Geometry check sheet. Reference: the model listing, model coordinates, mm. A direction names the side the tool comes from. Give positions to 0.01 mm unless a question says otherwise; leave off trailing zeros. Write each loop counter-clockwise with the first axis right and the second up, starting at its lowest first coordinate (ties: lowest second). Pieces come first, ordered by that corner, then holes. Notation, with made-up numbers: (-7, 62) -> (52, 62) arc R24 cw to (52, 80) -> close; hole circle Ø9 at (-7.75, 58). An arc over 180 degrees is marked (long way). One line per item, written item: value.
Autodesk Inventor part; units mm, degrees
ref_plane "YZ Plane" through (0, 0, 0) normal (1, 0, 0) x (0, 1, 0)
ref_plane "XZ Plane" through (0, 0, 0) normal (0, 1, 0) x (-1, 0, 0)
ref_plane "XY Plane" through (0, 0, 0) normal (0, 0, 1) x (1, 0, 0)
sketch "Sketch1" plane through (0, 0, 0) normal (0, 1, 0) x (-1, 0, 0)
  circle A0 centre (0, 0) radius 5
  dimension "d0" = 10
extrude "Extrusion1" add sketch "Sketch1" along normal blind 23
sketch "Sketch2" plane through (0, 23, 0) normal (0, 1, 0) x (1, 0, 0)
  line L0 (0, -4.5) -> (0, 4.5) construction
  circle A0 centre (0, 0) radius 5
  line L1 (-2.1794, -4.5) -> (2.1794, -4.5)
  line L2 (-2.1794, 4.5) -> (2.1794, 4.5)
extrude "Extrusion2" cut sketch "Sketch2" against normal blind 10 contours L2 A0 | A0 L1
sketch "Sketch3" plane through (0, 23, 0) normal (0, 1, 0) x (1, 0, 0)
  circle A0 centre (0, 0) radius 2.5
  dimension "d7" = 5
extrude "Extrusion3" add sketch "Sketch3" along normal blind 22
sketch "Sketch4" plane through (0, 0, 0) normal (0, -1, 0) x (1, 0, 0)
  circle A0 centre (0, 0) radius 2.5
  circle A1 centre (0, 0) radius 3
  dimension "d10" = 6
extrude "Extrusion4" add sketch "Sketch4" along normal blind 20 contours A0
thread "Thread1"
fillet "Fillet1" radius 0.5 1 edges at (-2.5, 45, 0)
thread "Thread2"
fillet "Fillet2" radius 0.5 1 edges at (-2.5, -20, 0)
properties part number "Semi alberto M"
1) Sectioned sample at B-B on z = 0. Record the cut outline in (x, y).
Verdict:
outline: (-5, 0) -> (-2.5, 0) -> (-2.5, -19.5) arc R0.5 ccw to (-2, -20) -> (2, -20) arc R0.5 ccw to (2.5, -19.5) -> (2.5, 0) -> (5, 0) -> (5, 23) -> (2.5, 23) -> (2.5, 44.5) arc R0.5 ccw to (2, 45) -> (-2, 45) arc R0.5 ccw to (-2.5, 44.5) -> (-2.5, 23) -> (-5, 23) -> close
2) Sectioned sample at C-C on y = 27. Record the cut outline in (x, z), plus the area to 3 significant figures.
Verdict:
outline: circle Ø5 at (0, 0)
area: 19.6 mm^2
3) Depth check by flat-ended pin: pin 1 Ø4 at (y, z) = (5, 3) entering from +X; pin 2 Ø1.3 at (x, y) = (0, 18) entering from -Z; pin 3 Ø2 at (y, z) = (10.5, 3.5) entering from -X. Enter the tip coordinate at first touch or a pass-through.
Verdict:
pin 1: x = 4.9
pin 2: z = -4.5
pin 3: x = -4.33
4) Tool access check on faces 1 (the flat face through (0, 18, 4.5)), 2 (the cylindrical face through (-4.619, 11.339, 1.915)), 3 (the flat face through (0, 18, -4.5)), 4 (the flat face through (2, 23, 2)), 5 (the cylindrical face through (-0.54, -9.61, 2.44)). Record the directions out of +Z, -Z, +X, -X, +Y, -Y that give a thin tool (end or side, any length) a straight path to the whole face; none if there is none.
Verdict:
face 1: +Z, +X, -X, +Y
face 2: +Y, -Y
face 3: -Z, +X, -X, +Y
face 4: +Y
face 5: -Y
5) Sectioned sample at A-A on x = 0. Record the cut outline in (y, z).
Verdict:
outline: (-20, -2) arc R0.5 ccw to (-19.5, -2.5) -> (0, -2.5) -> (0, -5) -> (13, -5) -> (13, -4.5) -> (23, -4.5) -> (23, -2.5) -> (44.5, -2.5) arc R0.5 ccw to (45, -2) -> (45, 2) arc R0.5 ccw to (44.5, 2.5) -> (23, 2.5) -> (23, 4.5) -> (13, 4.5) -> (13, 5) -> (0, 5) -> (0, 2.5) -> (-19.5, 2.5) arc R0.5 ccw to (-20, 2) -> close
6) Scan lines: probe 1 along Y at (x, z) = (0.25, 4.75); probe 2 along Y at (x, z) = (-4, -1); probe 3 along Z at (x, y) = (-0.75, 22). Record each from-to range of solid material in increasing order.
Verdict:
probe 1: 0 to 13
probe 2: 0 to 23
probe 3: -4.5 to 4.5
7) Sectioned sample at D-D on y = 5.5. Record the cut outline in (x, z).
Verdict:
outline: circle Ø10 at (0, 0)
